from build123d import *

# Parameters (mm, degrees)
F0_W      = 52.5
F0_H      = 72.5
F0_R      = 1.85
F1_DEPTH  = 10
F3_W      = 90
F3_H      = 10
F4_DEPTH  = 41
F5_R      = 2.25
F5_R_2    = 39
F7_DEPTH  = 89.0378417744
F9_W      = 80
F9_H      = 82
F8_W      = 80
F8_H      = 45
F11_R     = 39
F12_R     = 20
F15_DEPTH = 25


with BuildPart() as f1:
    # F0 (on Right) → F1 (new body)
    with BuildSketch(Plane.YZ):
        with Locations((0, 36.25)):
            Rectangle(F0_W, F0_H)
        with Locations((21.25, 7)):
            Circle(F0_R, mode=Mode.SUBTRACT)
        with Locations((-21.25, 45.5)):
            Circle(F0_R, mode=Mode.SUBTRACT)
    extrude(amount=F1_DEPTH)

    # F3 (on face) → F4 (join, symmetric)
    with BuildSketch(Plane(origin=(0, -11.7059208872, 6.7584165753), x_dir=(-1, 0, 0), z_dir=(0, 0.8660254038, -0.5))):
        with Locations((-45, 70.9118417744)):
            Rectangle(F3_W, F3_H)
    extrude(amount=F4_DEPTH, both=True)

    # F5 (on face) → F7 (cut, through all)
    with BuildSketch(Plane(origin=(0, 37.9559208872, 65.7415834247), x_dir=(1, 0, 0), z_dir=(0, 0.5, 0.8660254038))):
        with Locations((14, -49.5168331507)):
            Circle(F5_R)
        with Locations((86, -49.5168331507)):
            Circle(F5_R)
        with Locations((86, 22.4831668493)):
            Circle(F5_R)
        with Locations((14, 22.4831668493)):
            Circle(F5_R)
        with Locations((50, -13.5168331507)):
            Circle(F5_R_2)
    extrude(amount=-F7_DEPTH, mode=Mode.SUBTRACT)

    # F9 (on face) → F10 section 0
    with BuildSketch(Plane(origin=(0, 32.9559208872, 57.0813293868), x_dir=(1, 0, 0), z_dir=(0, -0.5, -0.8660254038))):
        with Locations((50, 13.5168331507)):
            Rectangle(F9_W, F9_H)
    # F8 (on offset) → F10 section 1
    with BuildSketch(Plane(origin=(0, 20.4559208872, 35.4306942922), x_dir=(1, 0, 0), z_dir=(0, -0.5, -0.8660254038))):
        with Locations((50, 13.5168331507)):
            Rectangle(F8_W, F8_H)
    loft()

    # F11 (on face) → F13 section 0
    with BuildSketch(Plane(origin=(0, 32.9559208872, 57.0813293868), x_dir=(1, 0, 0), z_dir=(0, -0.5, -0.8660254038))):
        with Locations((50, 13.5168331507)):
            Circle(F11_R)
    # F12 (on face) → F13 section 1
    with BuildSketch(Plane(origin=(0, 20.4559208872, 35.4306942922), x_dir=(1, 0, 0), z_dir=(0, -0.5, -0.8660254038))):
        with Locations((50, 13.5168331507)):
            Circle(F12_R)
    loft(mode=Mode.SUBTRACT)

    # F14 (on face) → F15 (cut, through all)
    with BuildSketch(Plane(origin=(0, 32.9559208872, 57.0813293868), x_dir=(1, 0, 0), z_dir=(0, -0.5, -0.8660254038))):
        with BuildLine():
            Line((10, 43.5168331507), (14, 43.5168331507))
            ThreePointArc((14, 43.5168331507), (18.2426406871, 45.2741924635), (20, 49.5168331507))
            Line((20, 49.5168331507), (20, 54.5168331507))
            Line((20, 54.5168331507), (10, 54.5168331507))
            Line((10, 54.5168331507), (10, 43.5168331507))
        make_face()
        with BuildLine():
            Line((9, -26.4831668493), (20, -26.4831668493))
            Line((20, -26.4831668493), (20, -22.4831668493))
            ThreePointArc((20, -22.4831668493), (18.2426406871, -18.2405261622), (14, -16.4831668493))
            Line((14, -16.4831668493), (9, -16.4831668493))
            Line((9, -16.4831668493), (9, -26.4831668493))
        make_face()
        with BuildLine():
            Line((90, -27.4831668493), (90, -16.4831668493))
            Line((90, -16.4831668493), (86, -16.4831668493))
            ThreePointArc((86, -16.4831668493), (81.7573593129, -18.2405261622), (80, -22.4831668493))
            Line((80, -22.4831668493), (80, -27.4831668493))
            Line((80, -27.4831668493), (90, -27.4831668493))
        make_face()
        with BuildLine():
            Line((91, 53.5168331507), (80, 53.5168331507))
            Line((80, 53.5168331507), (80, 49.5168331507))
            ThreePointArc((80, 49.5168331507), (81.7573593129, 45.2741924635), (86, 43.5168331507))
            Line((86, 43.5168331507), (91, 43.5168331507))
            Line((91, 43.5168331507), (91, 53.5168331507))
        make_face()
    extrude(amount=F15_DEPTH, mode=Mode.SUBTRACT)


solid = f1.part
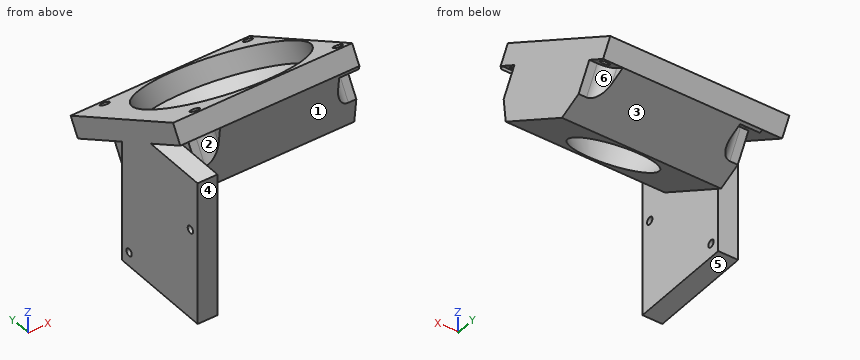
Input: part model. Units: mm. Frame: model coordinates. Face numbers are marked on the shaded views. A direction names the side the tool comes from. Round coordinates to 2 decimals unless told otherwise and drop trailing zeros. Order: outer loops, then holes, each group sorted by start corner. A loop starts at its lowest first (then second) coordinate and runs counter-clockwise, first axis right, second up.
1. Mould query, pull axis Y, two halves, no side actions, for the marked faces 4, 5 and 6. Classes: released by +Y, released by -Y, zero draft, split by the parting line, or undercut.
The answers:
face 4: released by -Y
face 5: zero draft
face 6: undercut
2. Set-up query: the marked faces 1, 2 and 3. Return all of +Z, -Z, +X, -X, +Y, -Y with unobstructed straight access to the full face (end or side cutting, diameter ignored); none if empty.
The answers:
face 1: -Z, +X, -Y
face 2: -Y
face 3: -Z, +X, -X, +Y
3. Cut plane B-B, the plane y = -21.25. Output: boundary loops of the cut face in (x, z), then the cut area to 3 significant figures.
The answers:
outline: (0, 0) - (10, 0) - (10, 43.65) - (0, 43.65) - close; (0, 47.35) - (10, 47.35) - (10, 72.5) - (0, 72.5) - close
area: 688 mm2
4. Material intervals for line 1 (Z direction, x = 2.75, y = -21.25); line 2 (Y direction, x = 4, z = 45); line 3 (X direction, y = 46.5, z = 53), sorted ascending.
The answers:
line 1: z = 0 to 43.65, 47.35 to 72.5
line 2: y = -26.25 to -23.03, -19.47 to 26.25, 53.88 to 57.72
line 3: x = 0 to 22.14, 77.86 to 90
5. Cut plane A-A, the plane z = 7. Output: boundary loops of the cut face in (x, y), then the cut area to 3 significant figures.
The answers:
outline: (0, -26.25) - (10, -26.25) - (10, 19.4) - (0, 19.4) - close; (0, 23.1) - (10, 23.1) - (10, 26.25) - (0, 26.25) - close
area: 488 mm2
6. Pin query (flat end, axial travel): P1, Ø1.8, axis at y = 51, z = 43.5, coming from the +X side; P2, Ø5, axis at x = 41, y = 23, coming from the -Z side; P3, Ø1.2, axis at y = -11.5, z = 81, coming from the +X side. Return the tip coordinate at first contact, or that it passes through.
The answers:
P1: stops at x = 80.08
P2: stops at z = 32.52
P3: stops at x = 80
